from build123d import *

# Parameters (mm, degrees)
SKETCH_1_R      = 17.5
SKETCH_1_R_2    = 1.5
EXTRUDE_1_DEPTH = 1
SKETCH_2_W      = 4.325123413
SKETCH_2_H      = 6.187329326
EXTRUDE_2_DEPTH = 1.2


with BuildPart() as part:
    # 草图1 → 凸台-拉伸1 (new body)
    with BuildSketch(Plane.XY):
        Circle(SKETCH_1_R)
        with Locations((0, 9.5)):
            Circle(SKETCH_1_R_2, mode=Mode.SUBTRACT)
        with Locations((0, -9.5)):
            Circle(SKETCH_1_R_2, mode=Mode.SUBTRACT)
        with Locations((10.606601718, 10.606601718)):
            Circle(SKETCH_1_R_2, mode=Mode.SUBTRACT)
        with Locations((10.606601718, -10.606601718)):
            Circle(SKETCH_1_R_2, mode=Mode.SUBTRACT)
        with Locations((-10.606601718, -10.606601718)):
            Circle(SKETCH_1_R_2, mode=Mode.SUBTRACT)
        with Locations((-10.606601718, 10.606601718)):
            Circle(SKETCH_1_R_2, mode=Mode.SUBTRACT)
    extrude(amount=EXTRUDE_1_DEPTH)

    # 草图2 → 凸台-拉伸2 (add)
    with BuildSketch(Plane.XY.offset(1)):
        with Locations((-0.090106737, 0.600711585)):
            Rectangle(SKETCH_2_W, SKETCH_2_H)
    extrude(amount=EXTRUDE_2_DEPTH)


solid = part.part
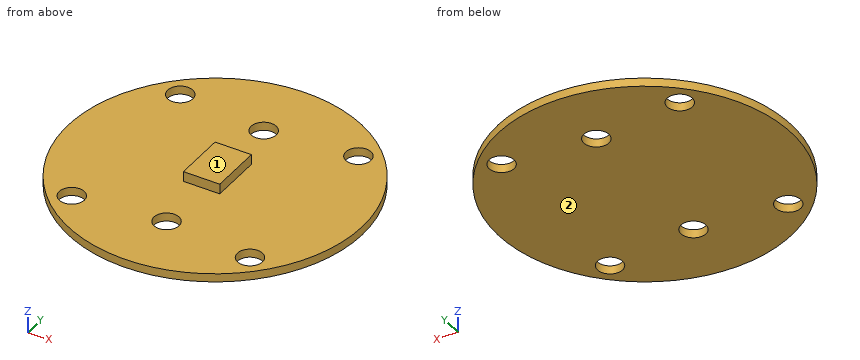
For this review, take the finished solid that the model builds, in its own axes (mm). Face numbers are marked on the shaded views. Give positions to 0.01 mm unless a question says otherwise; leave off trailing zeros. Loops run counter-clockwise (first coordinate to the right, second up) from the corner with the lowest first, then second, coordinate; pieces in that order, holes last. Notation, with made-up numbers: M 11.5,20.5 L 37.5,20.5 A35 ccw 37.5,56.5 Z; hole C 46,-8.75 d3. An arc over 180 degrees is marked long. Put each result on its own line as item: value. Start each with the question number.
(1) Add section D-D, the plane x = -10.5. Write out the cut boundary in (y, z).
(2) Add section C-C, the plane z = 1.85. Write out the cut boundary in (x, y).
(3) Add section B-B, the plane y = 0. Write out the cut boundary in (x, z).
(4) For pin 1 (2.5 mm diameter, centred on x = 10.61, y = 10.61, fed in from -Z); pin 2 (8 mm diameter, centred on x = 8, y = 11, fed in from -Z); pin 3 (5 mm diameter, centred on x = -10.61, y = 10.61, fed in from +Z); pin 4 (1.3 mm diameter, centred on x = 0.5, z = 2, fed in from +Y), all flat-tipped, find the tip position at first contact; note any pin that passes through.
(5) Add section A-A, the plane x = 0. Write out the cut boundary in (y, z).
(6) The part is to be moulded in two halves that separate along Z. For the marked faces 1 and 2, say which applies: +Z half, -Z half, draft (parallel to the pull), parting line (faces both ways), or undercut.
(7) Wall thickness on L1, parallel to Y at x = 0, z = 0.4; L2, parallel to Z at x = -7.5, y = -1; L3, parallel to Y at x = -1, z = 0.25: over which ranges is each line inside the solid? List them lowest first.
Result:
1. outline: M -14,0 L -12.1,0 L -12.1,1 L -14,1 Z; M -9.11,0 L 9.11,0 L 9.11,1 L -9.11,1 Z; M 12.1,0 L 14,0 L 14,1 L 12.1,1 Z
2. outline: M -2.25,-2.49 L 2.07,-2.49 L 2.07,3.69 L -2.25,3.69 Z
3. outline: M -17.5,0 L 17.5,0 L 17.5,1 L 2.07,1 L 2.07,2.2 L -2.25,2.2 L -2.25,1 L -17.5,1 Z
4. pin 1: passes through
4. pin 2: stops at z = 0
4. pin 3: stops at z = 1
4. pin 4: stops at y = 3.69
5. outline: M -17.5,0 L -11,0 L -11,1 L -17.5,1 Z; M -8,0 L 8,0 L 8,1 L 3.69,1 L 3.69,2.2 L -2.49,2.2 L -2.49,1 L -8,1 Z; M 11,0 L 17.5,0 L 17.5,1 L 11,1 Z
6. face 1: +Z half
6. face 2: -Z half
7. L1: y = -17.5 to -11, -8 to 8, 11 to 17.5
7. L2: z = 0 to 1
7. L3: y = -17.47 to -10.62, -8.38 to 8.38, 10.62 to 17.47
